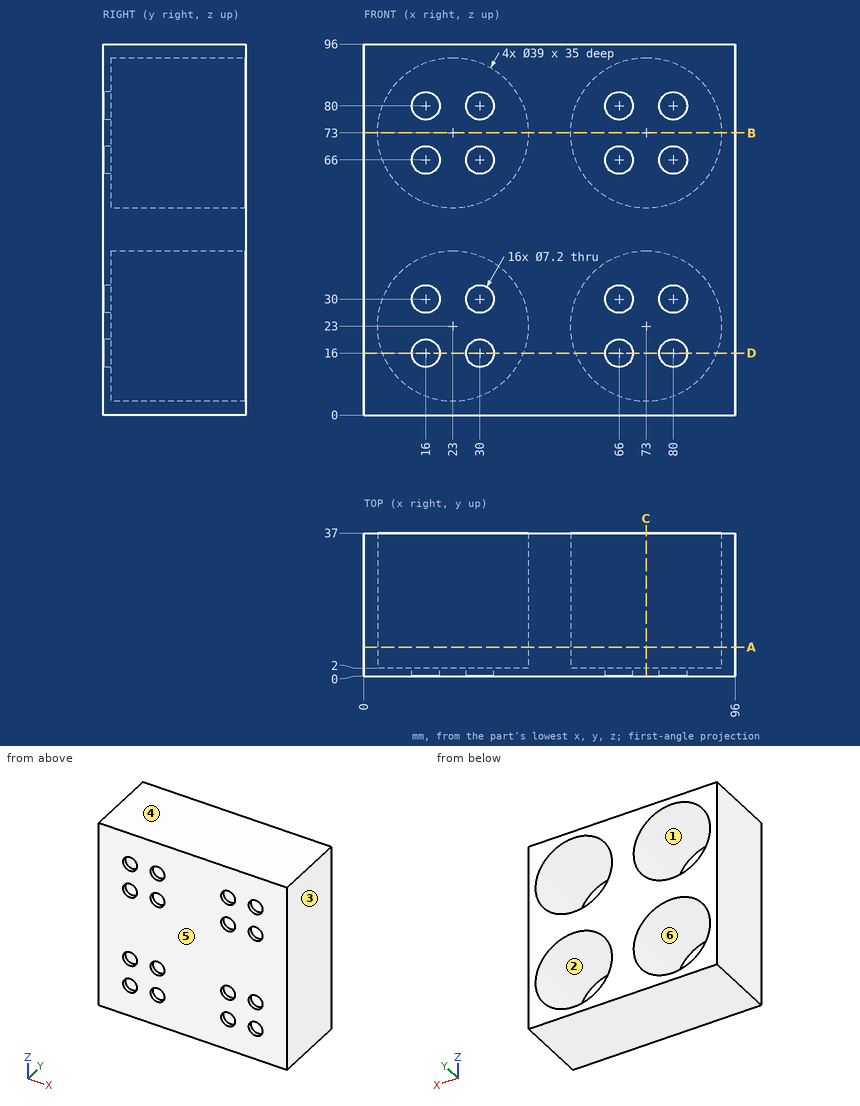
Verification items for this drawing (mm, ordinates from the low corner). A direction names the side the tool comes from. Give positions to 0.01 mm unless a question says otherwise; leave off trailing zeros. Write each loop counter-clockwise with the first axis right and the second up, starting at its lowest first coordinate (ties: lowest second). Pieces come first, ordered by that corner, then holes.
1) Material ranges on L1, parallel to X at y = 0.95, z = 16; L2, parallel to X at y = 16, z = 23.5; L3, parallel to X at y = 9.5, z = 58.5, recorded low to high.
2) Section check A-A, the plane y = 7.5. Record the boundary of the cut face in (x, z), and give its area (3 significant figures).
3) Section check B-B, the plane z = 73. Record the boundary of the cut face in (x, y), and give its area (3 significant figures).
4) Access from +Z, -Z, +X, -X, +Y, -Y to the whole of each face (thin tool, end or side, straight path). Record for the marked faces 5 and 6.
5) Gauge pin test, flat end, axial feed: pin 1 (2 mm diameter, centred on x = 12, z = 12, fed in from +Y). Record the tip position at first contact, or that the pin passes through.
6) Section check C-C, the plane x = 73. Record the boundary of the cut face in (y, z).
7) Release check for a two-part mould opening along X. For the marked faces 1, 2, 3 and 4 record: pulls with the +X half, pulls with the -X half, needs draft (parallel to the pull), parting line crosses it, or undercut.
8) Section check D-D, the plane z = 16. Record the boundary of the cut face in (x, y), and give its area (3 significant figures).
Computed:
1. L1: x = 0 to 12.4, 19.6 to 26.4, 33.6 to 62.4, 69.6 to 76.4, 83.6 to 96
1. L2: x = 0 to 3.51, 42.49 to 53.51, 92.49 to 96
1. L3: x = 0 to 9.96, 36.04 to 59.96, 86.04 to 96
2. outline: (0, 0) - (96, 0) - (96, 96) - (0, 96) - close; hole circle Ø39 at (23, 23); hole circle Ø39 at (23, 73); hole circle Ø39 at (73, 23); hole circle Ø39 at (73, 73)
2. area: 4,440 mm2
3. outline: (0, 0) - (96, 0) - (96, 37) - (92.5, 37) - (92.5, 2) - (53.5, 2) - (53.5, 37) - (42.5, 37) - (42.5, 2) - (3.5, 2) - (3.5, 37) - (0, 37) - close
3. area: 822 mm2
4. face 5: +Z, -Z, +X, -X, -Y
4. face 6: +Y
5. pin 1: stops at y = 2
6. outline: (0, 0) - (37, 0) - (37, 3.5) - (2, 3.5) - (2, 42.5) - (37, 42.5) - (37, 53.5) - (2, 53.5) - (2, 92.5) - (37, 92.5) - (37, 96) - (0, 96) - close
7. face 1: undercut
7. face 2: undercut
7. face 3: pulls with the +X half
7. face 4: needs draft
8. outline: (0, 0) - (12.4, 0) - (12.4, 2) - (4.8, 2) - (4.8, 37) - (0, 37) - close; (19.6, 0) - (26.4, 0) - (26.4, 2) - (19.6, 2) - close; (33.6, 0) - (62.4, 0) - (62.4, 2) - (54.8, 2) - (54.8, 37) - (41.2, 37) - (41.2, 2) - (33.6, 2) - close; (69.6, 0) - (76.4, 0) - (76.4, 2) - (69.6, 2) - close; (83.6, 0) - (96, 0) - (96, 37) - (91.2, 37) - (91.2, 2) - (83.6, 2) - close
8. area: 946 mm2
